from build123d import *

# Parameters (mm, degrees)
RESSALTO_EXTRUS_O1_DEPTH = 9.525
ESBO_O3_R                = 2.5
CORTE_EXTRUS_O1_DEPTH    = 23
ESBO_O11_R               = 2.78
CORTE_EXTRUS_O4_DEPTH    = 9.525
ESBO_O13_R               = 17
CORTE_EXTRUS_O5_DEPTH    = 10
ESBO_O14_R               = 2.78
CORTE_EXTRUS_O6_DEPTH    = 9.525
ESBO_O16_R               = 4.75
CORTE_EXTRUS_O9_DEPTH    = 3


with BuildPart() as part:
    # Esboço2 → Ressalto-extrusão1 (new body)
    with BuildSketch(Plane.XY):
        Polygon((-40, 35), (-40, 0), (-40, -35), (40, -35), (40, 0), (40, 35), align=None)
    extrude(amount=RESSALTO_EXTRUS_O1_DEPTH)

    # Esboço3 → Corte-extrusão1 (cut)
    with BuildSketch(Plane(origin=(0, 35, 0), x_dir=(-1, 0, 0), z_dir=(0, 1, 0))):
        with Locations((20, 4.7625)):
            Circle(ESBO_O3_R)
        with Locations((0, 4.7625)):
            Circle(ESBO_O3_R)
        with Locations((-20, 4.7625)):
            Circle(ESBO_O3_R)
    extrude(amount=-CORTE_EXTRUS_O1_DEPTH, mode=Mode.SUBTRACT)

    # Esboço11 → Corte-extrusão4 (cut)
    with BuildSketch(Plane.XY.offset(9.525)):
        with Locations((-20, -30.2375)):
            Circle(ESBO_O11_R)
        with Locations((20, -30)):
            Circle(ESBO_O11_R)
    extrude(amount=-CORTE_EXTRUS_O4_DEPTH, mode=Mode.SUBTRACT)

    # Esboço13 → Corte-extrusão5 (cut)
    with BuildSketch(Plane(origin=(0, 0, 0), x_dir=(-1, 0, 0), z_dir=(0, 0, -1))):
        with Locations((0, 5)):
            Circle(ESBO_O13_R)
    extrude(amount=-CORTE_EXTRUS_O5_DEPTH, mode=Mode.SUBTRACT)

    # Esboço14 → Corte-extrusão6 (cut)
    with BuildSketch(Plane(origin=(0, 0, 0), x_dir=(-1, 0, 0), z_dir=(0, 0, -1))):
        with Locations((-23.015, 5)):
            Circle(ESBO_O14_R)
        with Locations((-11.5075, -15)):
            Circle(ESBO_O14_R)
        with Locations((-11.5075, 25)):
            Circle(ESBO_O14_R)
        with Locations((11.428624391, 25)):
            Circle(ESBO_O14_R)
        with Locations((22.936124391, 5)):
            Circle(ESBO_O14_R)
        with Locations((11.428624391, -15)):
            Circle(ESBO_O14_R)
    extrude(amount=-CORTE_EXTRUS_O6_DEPTH, mode=Mode.SUBTRACT)

    # Esboço16 → Corte-extrusão9 (cut)
    with BuildSketch(Plane.XY.offset(9.525)):
        with Locations((-22.936124391, 5)):
            Circle(ESBO_O16_R)
        with Locations((-11.428624391, 25)):
            Circle(ESBO_O16_R)
        with Locations((11.5075, 25)):
            Circle(ESBO_O16_R)
        with Locations((23.015, 5)):
            Circle(ESBO_O16_R)
        with Locations((11.5075, -15)):
            Circle(ESBO_O16_R)
        with Locations((-11.428624391, -15)):
            Circle(ESBO_O16_R)
    extrude(amount=-CORTE_EXTRUS_O9_DEPTH, mode=Mode.SUBTRACT)


solid = part.part
Could you check a few things on this model? Use its own coordinates, in mm. A direction names the side the tool comes from. Give positions to 0.01 mm unless a question says otherwise; leave off trailing zeros. Loops run counter-clockwise (first coordinate to the right, second up) from the corner with the lowest first, then second, coordinate; pieces in that order, holes last. Notation, with made-up numbers: (-32, -36) -> (-19, -36) arc R22 ccw to (-19, -13) -> close; hole circle Ø6 at (-25.75, 22). An arc over 180 degrees is marked (long way). Answer as CSV lines item,"result". Start each with the question number.
(1) I need wall thicknesses on probe 1 along X at (y, z) = (-15.5, 3.75); probe 2 along Y at (x, z) = (-21, 7.5); probe 3 along Y at (x, z) = (9, 1). Which ranges of each line are inside material? Lowest first, please.
(2) Which directions (+Z, -Z, +X, -X, +Y, -Y) give clear straight access to the entire face, cutting with the end or side of a thin tool? Please do faces 4 (the cylindrical face through (-17.502, 23.661, 4.872)), 5 (the cylindrical face through (13.556, 26.879, 3.217)), 6 (the flat face through (26, 5, 6.525)).
(3) If we section it at C-C on y = 5: Write out the boundary of the cut face in (x, z) (3 decimals), then the cut area to 3 significant figures.
(4) If we section it at D-D on z = 3.75: Count the separate pieces of the cut face and the enclosed holes in it, then the cut area to 3 significant figures.
(5) I'm going to push flat-ended pins straight in: pin 1 Ø6.5 at (x, y) = (23.015, 5) entering from +Z (3 decimals); pin 2 Ø12.5 at (x, y) = (23.015, 5) entering from -Z; pin 3 Ø2.5 at (x, z) = (-19.5, 5.5) entering from +Y; pin 4 Ø4.5 at (x, z) = (0, 4.76) entering from +Y. Where does each tip first touch, or does it pass through?
(6) If we section it at B-B on x = 0: Write out the boundary of the cut face in (y, z) (1 decimal), then the cut area to 3 significant figures.
(7) We'd pull the mould along Z, two halves only. Please class faces 1 (the cylindrical face through (-12.05, 29.71, 8.05)), 2 (the cylindrical face through (22.498, 23.661, 4.872)), 3 (the flat face through (-1, -15, 0)): released by +Z, released by -Z, zero draft, split by the parting line, or undercut.
(8) If we section it at A-A on y = -15: Write out the boundary of the cut face in (x, z) (1 decimal).
Computed:
1,probe 1,"x = -40 to -14.16, -8.69 to 8.77, 14.24 to 40"
1,probe 2,"y = -35 to -32.83, -27.64 to 0.66, 9.34 to 35"
1,probe 3,"y = -35 to -16.2, -13.8 to -9.42, 19.42 to 23.8, 26.2 to 35"
2,face 4,"+Y"
2,face 5,"+Z, -Z"
2,face 6,"+Z"
3,outline,"(-40, 0) -> (-25.716, 0) -> (-25.716, 6.525) -> (-27.686, 6.525) -> (-27.686, 9.525) -> (-40, 9.525) -> close; (-20.156, 0) -> (-17, 0) -> (-17, 9.525) -> (-18.186, 9.525) -> (-18.186, 6.525) -> (-20.156, 6.525) -> close; (17, 0) -> (20.235, 0) -> (20.235, 6.525) -> (18.265, 6.525) -> (18.265, 9.525) -> (17, 9.525) -> close; (25.795, 0) -> (40, 0) -> (40, 9.525) -> (27.765, 9.525) -> (27.765, 6.525) -> (25.795, 6.525) -> close"
3,area,"309 mm2"
4,separate pieces,"1"
4,enclosed holes,"8"
4,area,"4,230 mm2"
5,pin 1,"stops at z = 6.525"
5,pin 2,"stops at z = 0"
5,pin 3,"stops at y = 12"
5,pin 4,"stops at y = -11.85"
6,outline,"(-35, 0) -> (-12, 0) -> (-12, 9.5) -> (-35, 9.5) -> close; (22, 0) -> (35, 0) -> (35, 2.3) -> (22, 2.3) -> close; (22, 7.3) -> (35, 7.3) -> (35, 9.5) -> (22, 9.5) -> close"
6,area,"278 mm2"
7,face 1,"zero draft"
7,face 2,"undercut"
7,face 3,"released by -Z"
8,outline,"(-40, 0) -> (-14.2, 0) -> (-14.2, 6.5) -> (-16.2, 6.5) -> (-16.2, 9.5) -> (-40, 9.5) -> close; (-8.6, 0) -> (8.7, 0) -> (8.7, 6.5) -> (6.8, 6.5) -> (6.8, 9.5) -> (-6.7, 9.5) -> (-6.7, 6.5) -> (-8.6, 6.5) -> close; (14.3, 0) -> (40, 0) -> (40, 9.5) -> (16.3, 9.5) -> (16.3, 6.5) -> (14.3, 6.5) -> close"
